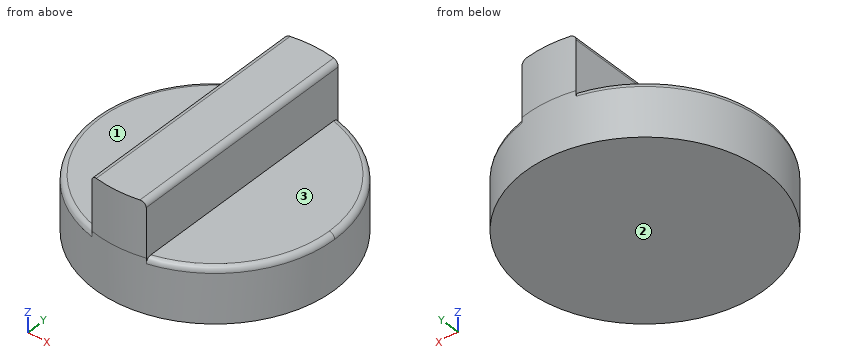
```python
from build123d import *

# Parameters (mm, degrees)
ESQUISSE1_R        = 11
BOSS_EXTRU_1_DEPTH = 5
BOSS_EXTRU_2_DEPTH = 5
CONG_1_R           = 0.5
CONG_2_R           = 0.5


with BuildPart() as part:
    # Esquisse1 → Boss.-Extru.1 (new body)
    with BuildSketch(Plane.XY):
        Circle(ESQUISSE1_R)
    extrude(amount=BOSS_EXTRU_1_DEPTH)

    # Esquisse2 → Boss.-Extru.2 (add)
    with BuildSketch(Plane.XY.offset(5)):
        with BuildLine():
            Line((-2.5, 10.712142643), (-2.5, -10.712142643))
            ThreePointArc((-2.5, -10.712142643), (0, -11), (2.5, -10.712142643))
            Line((2.5, -10.712142643), (2.5, 10.712142643))
            ThreePointArc((2.5, 10.712142643), (0, 11), (-2.5, 10.712142643))
        make_face()
    extrude(amount=BOSS_EXTRU_2_DEPTH)

    # Congé1
    # the kernel refuses this fillet: 0.5 mm, written as the material it takes off along each edge
    with BuildSketch(Plane(origin=(0, 0, 5), x_dir=(1, 0, 0), z_dir=(0, -1, 0))) as cong_1_piece_1_section:
        with BuildLine():
            CenterArc((11 - CONG_1_R, -CONG_1_R), CONG_1_R, 0, 90)
            Line((11 - CONG_1_R, 0), (11, 0))
            Line((11, 0), (11, -CONG_1_R))
        make_face()
    cong_1_piece_1 = revolve(axis=Axis((0, 0, 5), (0, 0, 1)), revolution_arc=83.376232782, mode=Mode.PRIVATE)
    cong_1_piece_1 = split(cong_1_piece_1, bisect_by=Plane(origin=(2.5, 6.750657891, 4.860453912), z_dir=(1, 0, 0)), keep=Keep.TOP, mode=Mode.PRIVATE)
    add(cong_1_piece_1, mode=Mode.SUBTRACT)
    with BuildSketch(Plane(origin=(0, 0, 5), x_dir=(-0.11524991416990704, 0.9933365277104376, 0), z_dir=(0.9933365277104376, 0.11524991416990704, 0))) as cong_1_piece_2_section:
        with BuildLine():
            CenterArc((11 - CONG_1_R, -CONG_1_R), CONG_1_R, 0, 90)
            Line((11 - CONG_1_R, 0), (11, 0))
            Line((11, 0), (11, -CONG_1_R))
        make_face()
    cong_1_piece_2 = revolve(axis=Axis((0, 0, 5), (0, 0, 1)), revolution_arc=166.76392016, mode=Mode.PRIVATE)
    cong_1_piece_2 = split(cong_1_piece_2, bisect_by=Plane(origin=(-2.5, 0, 4.862247452), z_dir=(-1, 0, 0)), keep=Keep.TOP, mode=Mode.PRIVATE)
    add(cong_1_piece_2, mode=Mode.SUBTRACT)
    with BuildSketch(Plane(origin=(0, 0, 5), x_dir=(0.1153492077124676, -0.9933250023431938, 0), z_dir=(-0.9933250023431938, -0.1153492077124676, 0))) as cong_1_piece_3_section:
        with BuildLine():
            CenterArc((11 - CONG_1_R, -CONG_1_R), CONG_1_R, 0, 90)
            Line((11 - CONG_1_R, 0), (11, 0))
            Line((11, 0), (11, -CONG_1_R))
        make_face()
    cong_1_piece_3 = revolve(axis=Axis((0, 0, 5), (0, 0, 1)), revolution_arc=83.376232782, mode=Mode.PRIVATE)
    cong_1_piece_3 = split(cong_1_piece_3, bisect_by=Plane(origin=(2.5, -6.750657902, 4.860453931), z_dir=(1, 0, 0)), keep=Keep.TOP, mode=Mode.PRIVATE)
    add(cong_1_piece_3, mode=Mode.SUBTRACT)

    # Congé2
    cong_2_edges = [part.edges().sort_by_distance(p)[0] for p in [
        (-2.5, 0, 10),
        (2.5, 0, 10),
    ]]
    fillet(cong_2_edges, radius=CONG_2_R)


solid = part.part
```
The listing builds one solid part. Answer for the finished solid, in the listing's coordinates (mm). Face numbers are marked on the shaded views. A direction names the side the tool comes from. Give positions to 0.01 mm unless a question says otherwise; leave off trailing zeros. Order: outer loops, then holes, each group sorted by start corner. A loop starts at its lowest first (then second) coordinate and runs counter-clockwise, first axis right, second up. Notation, with made-up numbers: (50.25, 37) -> (95.25, 37) arc R34 cw to (95.25, 76) -> close; hole circle Ø5 at (-26, -26). An arc over 180 degrees is marked (long way). Answer as a JSON object with one key per item and string values. Group by question number.
Item 1: Flat-ended cylindrical pins translate along their axes: pin 1 (1.5 mm diameter, centred on x = 1.5, z = 6, fed in from +Y); pin 2 (5.5 mm diameter, centred on y = 1.5, z = 8, fed in from -X); pin 3 (1.5 mm diameter, centred on y = 5.5, z = 6.5, fed in from +X). Find the tip coordinate at first contact, or state that the pin passes through.
Item 2: The part is cut by section B-B on z = 2.5. Write down the section's boundary in (x, y).
Item 3: A tool of negligible diameter and unlimited length cuts with its end or side. For the marked faces 1, 2 and 3, from which of +Z, -Z, +X, -X, +Y, -Y can it reach the whole face along a straight path? Write none if from no direction.
Item 4: Consider L1, parallel to X at y = 6.5, z = 7.5; L2, parallel to X at y = -2, z = 4.25; L3, parallel to Z at x = -9.75, y = 3.25. Determine where each line is inside the solid, lowest interval first. Write a range as from..to.
Item 5: The part is cut by section A-A on z = 7.5. Write down the section's boundary in (x, y).
Result set:
{
 "1": {"pin 1": "y = 10.97", "pin 2": "x = -2.5", "pin 3": "x = 2.5"},
 "2": {"outline": "circle Ø22 at (0, 0)"},
 "3": {"face 1": "+Z, -X, +Y, -Y", "face 2": "-Z, +X, -X, +Y, -Y", "face 3": "+Z, +X, +Y, -Y"},
 "4": {"L1": "-2.5..2.5", "L2": "-10.82..10.82", "L3": "0..5"},
 "5": {"outline": "(-2.5, -10.71) arc R11 ccw to (2.5, -10.71) -> (2.5, 10.71) arc R11 ccw to (-2.5, 10.71) -> close"}
}
